Source: CAD feature listing. Evaluate the final solid. Frame: model axes, mm. A direction names the side the tool comes from. Coordinates: 2 decimals unless noted, no trailing zeros. Write each loop counter-clockwise with the first axis right and the second up, starting at its lowest first coordinate (ties: lowest second). Pieces come first, ordered by that corner, then holes. Notation, with made-up numbers: M 20,5 L 39,5 A22 cw 39,32 Z; hole C 38.25,24 d8. An arc over 180 degrees is marked long. Write item = value, one per line. Start each with the question number.
1. Pull-direction query (X, two-part tool) for faces 3 (the face through (0, 31, 285)), 4 (the face through (30, 10.197, 375)), 5 (the face through (59.995, 31, 285)); classes: pulls with the +X half, pulls with the -X half, needs draft (parallel to the pull), parting line crosses it, or undercut.
2. Pin query (flat end, axial travel): pin 1 Ø4 at (y, z) = (17, 67) entering from -X. Return the tip coordinate at first contact, or that it passes through.
3. Line query: line 1 along Z through (x, y) = (33.5, 40.5); line 2 along Z through (x, y) = (30, 21.5); line 3 along Z through (x, y) = (26, 58.5). Output: solid intervals per line, ascending.
4. Section query B-B (x = 37.5). Output: boundary loops of the cut face in (y, z), then the cut area to 3 significant figures.
5. Section query A-A (y = 25). Output: boundary loops of the cut face in (x, z), then the cut area to 3 significant figures.
6. Access query for faces 1 (the face through (30.417, 57.178, -15.345)), 2 (the face through (43.6, 36, 354.4)). Directions: +Z, -Z, +X, -X, +Y, -Y. A direction counts if a zero-diameter tool reaches every point of the face in a straight line with its end or side. Return the directions, or none.
7. Section query C-C (z = 515). Output: boundary loops of the cut face in (x, y).
Autodesk Inventor part; units mm, degrees
ref_plane "YZ Plane" through (0, 0, 0) normal (1, 0, 0) x (0, 1, 0)
ref_plane "XZ Plane" through (0, 0, 0) normal (0, 1, 0) x (-1, 0, 0)
ref_plane "XY Plane" through (0, 0, 0) normal (0, 0, 1) x (1, 0, 0)
sketch "Sketch1" plane through (0, 0, 0) normal (1, 0, 0) x (0, 1, 0)
  line L0 (0.9972, 8.0994) -> (0.9972, -18.9664)
  line L1 (0.9972, -18.9664) -> (0.9972, 581.0324)
  line L2 (0.9972, 581.0324) -> (60.997, 581.0324)
  line L3 (60.997, 581.0324) -> (60.997, -18.9664)
  line L4 (60.997, -18.9664) -> (0.9972, -18.9664)
  point P0 (0, 0)
  dimension "d0" = 599.9988
  dimension "d1" = 59.9999
extrude "Extrusion1" add sketch "Sketch1" along normal blind 59.9948
sketch "Sketch2" plane through (59.9948, 0, 0) normal (1, 0, 0) x (0, 0, -1)
  circle A0 centre (-525.9231, 30.9971) radius 25.4
  circle A1 centre (-45.3472, 30.9971) radius 25.4
  point P0 (0, 0)
  dimension "d4" = 50.8
  dimension "d5" = 50.8
extrude "Extrusion2" cut sketch "Sketch2" against normal blind 59.9948
fillet "Fillet1" radius 12.7 4 edges at (29.9974, 60.997, 581.0324) (29.9974, 0.9972, 581.0324) (29.9974, 60.997, -18.9664) (29.9974, 0.9972, -18.9664)
sketch "Sketch3" plane through (0, 60.997, 568.3324) normal (0, 1, 0) x (1, 0, 0)
  circle A0 centre (29.9562, 192.5093) radius 25.4
  point P0 (0, 568.3324)
  dimension "d9" = 50.8
extrude "Extrusion3" cut sketch "Sketch3" against normal blind 50.8
properties part number "legrod" material "Wood (Birch)"
Results are:
q1.face_3 = pulls with the -X half
q1.face_4 = undercut
q1.face_5 = pulls with the +X half
q2.pin_1 = 0
q3.line_1 = -18.97 to 21.79, 68.9 to 350.67, 400.97 to 502.37, 549.48 to 581.03
q3.line_2 = -18.97 to 21.79, 68.9 to 350.42, 401.22 to 502.37, 549.48 to 581.03
q3.line_3 = -13.83 to 350.73, 400.91 to 575.89
q4.outline = M 1,-6.27 A12.7 ccw 13.7,-18.97 L 48.3,-18.97 A12.7 ccw 61,-6.27 L 61,351.57 L 10.2,351.57 L 10.2,400.08 L 61,400.08 L 61,568.33 A12.7 ccw 48.3,581.03 L 13.7,581.03 A12.7 ccw 1,568.33 Z; hole C 31,45.35 d50.8; hole C 31,525.92 d50.8
q4.area = 29,300 mm^2
q5.outline = M 0,-18.97 L 59.99,-18.97 L 59.99,20.67 L 0,20.67 Z; M 0,70.03 L 59.99,70.03 L 59.99,501.24 L 0,501.24 Z; M 0,550.6 L 59.99,550.6 L 59.99,581.03 L 0,581.03 Z; hole C 29.96,375.82 d50.8
q5.area = 28,000 mm^2
q6.face_1 = -Z, +X, -X, +Y
q6.face_2 = +Y
q7.outline = M 0,1 L 59.99,1 L 59.99,8.07 L 0,8.07 Z; M 0,53.93 L 59.99,53.93 L 59.99,61 L 0,61 Z
